Input: part model. Units: mm. Frame: model coordinates. Face numbers are marked on the shaded views. Round coordinates to 2 decimals unless told otherwise and drop trailing zeros. Write each loop counter-clockwise with the first axis right and the second up, starting at its lowest first coordinate (ties: lowest second). Pieces come first, ordered by that corner, then holes. Notation, with made-up numbers: (60, -18) -> (100, -18) arc R22 ccw to (100, -7) -> close; hole circle Ø3 at (15.5, -11). An arc over 180 degrees is marked (long way). Write item = value, one per line.
```python
from build123d import *

# Parameters (mm, degrees)
SKETCH1_W           = 57.15
SKETCH1_H           = 57.15
BOSS_EXTRUDE1_DEPTH = 19.05
SKETCH2_R           = 19.2405
CUT_EXTRUDE1_DEPTH  = 19.05
SKETCH5_R           = 3.175
CUT_EXTRUDE2_DEPTH  = 84.037024874
SKETCH6_R           = 3.175
CUT_EXTRUDE3_DEPTH  = 84.037024966


with BuildPart() as part:
    # Sketch1 → Boss-Extrude1 (new body)
    with BuildSketch(Plane.XY):
        with Locations((28.575, 28.575)):
            Rectangle(SKETCH1_W, SKETCH1_H)
    extrude(amount=BOSS_EXTRUDE1_DEPTH)

    # Sketch2 → Cut-Extrude1 (cut)
    with BuildSketch(Plane(origin=(0, 0, 0), x_dir=(-1, 0, 0), z_dir=(0, 0, -1))):
        with Locations((-28.575, 28.575)):
            Circle(SKETCH2_R)
    extrude(amount=-CUT_EXTRUDE1_DEPTH, mode=Mode.SUBTRACT)

    # Sketch5 → Cut-Extrude2 (cut, through all)
    with BuildSketch(Plane(origin=(57.15, 0, 0), x_dir=(0, 0, -1), z_dir=(1, 0, 0))):
        with Locations((-9.525, 28.575)):
            Circle(SKETCH5_R)
    extrude(amount=-CUT_EXTRUDE2_DEPTH, mode=Mode.SUBTRACT)

    # Sketch6 → Cut-Extrude3 (cut, through all)
    with BuildSketch(Plane.XZ):
        with Locations(Location((28.575, 9.525, 0), (0, 0, 270))):
            Circle(SKETCH6_R)
    extrude(amount=-CUT_EXTRUDE3_DEPTH, mode=Mode.SUBTRACT)


solid = part.part
```
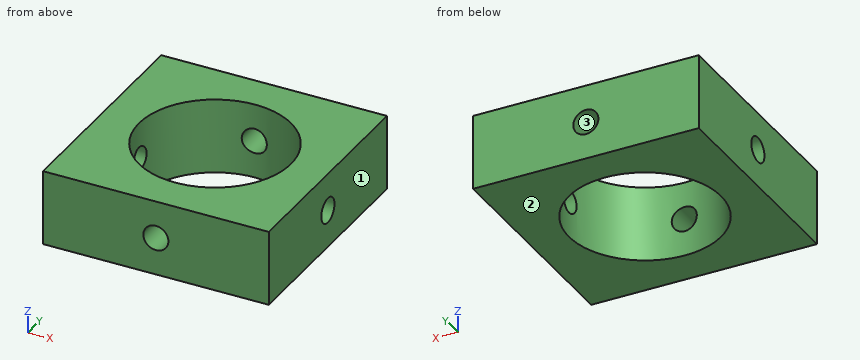
1) Cut plane A-A (y = 35). Return the cut outline in (x, z).
Solutions:
outline = (0, 0) -> (10.44, 0) -> (10.44, 19.05) -> (0, 19.05) -> close; (46.71, 0) -> (57.15, 0) -> (57.15, 19.05) -> (46.71, 19.05) -> close
2) Line query: L1, parallel to X at y = 29, z = 1.5; L2, parallel to Y at x = 28.5, z = 15; L3, parallel to X at y = 48.5, z = 7.5. Output: solid intervals per line, ascending. Write a range as from..to.
Solutions:
L1 = 0..9.34, 47.81..57.15
L2 = 0..9.33, 47.82..57.15
L3 = 0..26.13, 31.02..57.15
3) Cut plane D-D (x = 27). Return the cut outline in (y, z), and give its area (3 significant figures).
Solutions:
outline = (0, 0) -> (9.4, 0) -> (9.4, 6.77) -> (0, 6.77) -> close; (0, 12.28) -> (9.4, 12.28) -> (9.4, 19.05) -> (0, 19.05) -> close; (47.75, 0) -> (57.15, 0) -> (57.15, 6.77) -> (47.75, 6.77) -> close; (47.75, 12.28) -> (57.15, 12.28) -> (57.15, 19.05) -> (47.75, 19.05) -> close
area = 254 mm^2
4) Cut plane C-C (x = 44.5). Return the cut outline in (y, z), and give its area (3 significant figures).
Solutions:
outline = (0, 0) -> (17.78, 0) -> (17.78, 19.05) -> (0, 19.05) -> close; (39.37, 0) -> (57.15, 0) -> (57.15, 19.05) -> (39.37, 19.05) -> close
area = 677 mm^2
5) Draft query along X for the marked faces 1, 2 and 3. Return one class per face: +X half, -X half, draft (parallel to the pull), parting line (faces both ways), or undercut.
Solutions:
face_1 = +X half
face_2 = draft
face_3 = undercut
6) Cut plane B-B (z = 11.75). Count the separate pieces of the cut face and the enclosed holes in it, and give its area (3 significant figures).
Solutions:
separate_pieces = 4
enclosed_holes = 0
area = 1,930 mm^2
